Read the model definition and answer for the solid it produces. Units are mm, in the model's axes. Face numbers are marked on the shaded views. A direction names the side the tool comes from. Coordinates: 2 decimals unless noted, no trailing zeros. Write each loop counter-clockwise with the first axis right and the second up, starting at its lowest first coordinate (ties: lowest second). Pieces come first, ordered by that corner, then holes. Notation, with made-up numbers: M 83.5,-3.5 L 131.5,-3.5 A28 ccw 131.5,32.5 Z; hole C 41,87 d8. An arc over 180 degrees is marked long. Write item = value, one per line.
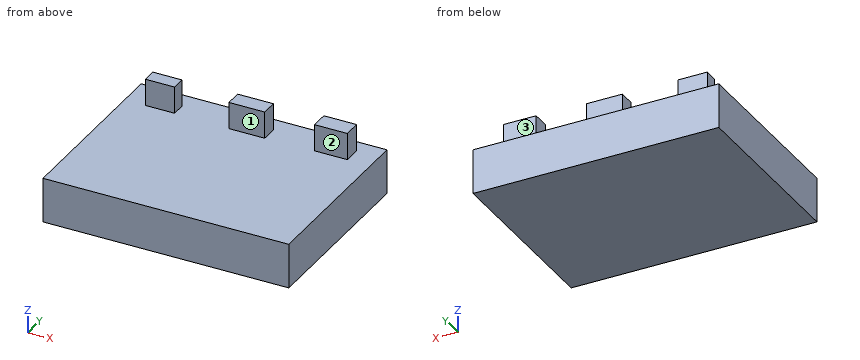
from build123d import *

# Parameters (mm, degrees)
F0_W     = 54.88
F0_H     = 41.5
F1_DEPTH = 10
F2_W     = 6.537087
F2_H     = 3.137803
F2_W_2   = 7.990626
F2_H_2   = 3.66077
F2_W_3   = 7.32154
F2_H_3   = 3.92225
F3_DEPTH = 6


with BuildPart() as f1:
    # F0 (on Top) → F1 (new body)
    with BuildSketch(Plane.XY):
        Rectangle(F0_W, F0_H)
    extrude(amount=F1_DEPTH)

    # F2 (on face) → F3 (join)
    with BuildSketch(Plane.XY.offset(10)):
        with Locations((-19.538203, 15.287418)):
            Rectangle(F2_W, F2_H)
        with Locations((0, 15.287419)):
            Rectangle(F2_W_2, F2_H_2)
        with Locations((18.638391, 15.679644)):
            Rectangle(F2_W_3, F2_H_3)
    extrude(amount=F3_DEPTH)


solid = f1.part
Item 1: Consider line 1 along Z through (x, y) = (-7.5, 7). Determine where the line is inside the solid, lowest interval first. Write a range as from..to.
Worked answers:
line_1 = 0..10
Item 2: Find section B-B (x = -19). Determine the outline of the cut face in (y, z), and give its area (3 significant figures).
Worked answers:
outline = M -20.75,0 L 20.75,0 L 20.75,10 L 16.86,10 L 16.86,16 L 13.72,16 L 13.72,10 L -20.75,10 Z
area = 434 mm²
Item 3: Find section D-D (x = 20). Determine the outline of the cut face in (y, z), and give its area (3 significant figures).
Worked answers:
outline = M -20.75,0 L 20.75,0 L 20.75,10 L 17.64,10 L 17.64,16 L 13.72,16 L 13.72,10 L -20.75,10 Z
area = 439 mm²
Item 4: Find section C-C (y = -7). Determine the outline of the cut face in (x, z).
Worked answers:
outline = M -27.44,0 L 27.44,0 L 27.44,10 L -27.44,10 Z
Item 5: Flat-ended cylindrical pins translate along their axes: pin 1 (1.6 mm diameter, centred on y = 15.5, z = 13.5, fed in from +X); pin 2 (5 mm diameter, centred on x = -2, z = 14.5, fed in from -Y); pin 3 (21 mm diameter, centred on x = -12, y = 3, fed in from +Z). Find the tip coordinate at first contact, or state that the pin passes through.
Worked answers:
pin_1 = 22.3
pin_2 = 13.46
pin_3 = 10
Item 6: Which of the six approach directions +Z, -Z, +X, -X, +Y, -Y give full straight-line access (tool end or side, diameter ignored) to the marked faces 1, 2 and 3?
Worked answers:
face_1 = +Z, +X, -X, -Y
face_2 = +Z, +X, -Y
face_3 = +Z, +X, -X, +Y
Item 7: Find section A-A (z = 12.5). Determine the outline of the cut face in (x, y), and give its area (3 significant figures).
Worked answers:
outline = M -22.81,13.72 L -16.27,13.72 L -16.27,16.86 L -22.81,16.86 Z; M -4,13.46 L 4,13.46 L 4,17.12 L -4,17.12 Z; M 14.98,13.72 L 22.3,13.72 L 22.3,17.64 L 14.98,17.64 Z
area = 78.5 mm²
